Check sheet for the drawn part. Datum: minimum x, y, z corner. Units: mm. A direction names the side the tool comes from. Coordinates: 2 decimals unless noted, no trailing zeros. Order: outer loops, then holes, each group sorted by start corner. A loop starts at its lowest first (then second) coordinate and runs counter-clockwise, first axis right, second up. Notation, with made-up numbers: (12.5, -24) - (64.5, -24) arc R24 cw to (64.5, -11) - close; hole circle Ø2 at (25, 77). An arc over 180 degrees is marked (long way). Answer as CSV lines item,"result". Start each with the question number.
1. Section check A-A (y = 4.9). Record the cut outline in (x, z).
2. Mould release check, pull along Z, two halves, no side actions. Record for the marked faces 4, 5 and 6: pulls with the +Z half, pulls with the -Z half, needs draft (parallel to the pull), parting line crosses it, or undercut.
3. Material ranges on L1, parallel to Z at x = 6.5, y = 4.35; L2, parallel to Z at x = 5.5, y = 5.1; L3, parallel to Z at x = 6.5, y = 3.85, recorded low to high. Write a range as [from, to].
4. Go/stop test with a flat-tipped pin: pin 1 (2.5 mm diameter, centred on x = 7, z = 8, fed in from -Y). Record where the tip stops, or that it passes through.
5. Set-up check for the marked faces 1, 2 and 3: record each of +Z, -Z, +X, -X, +Y, -Y from which the full face is reachable in a straight line by a thin tool's end or side.
6. Section check D-D (x = 6.5). Record the cut outline in (y, z).
7. Section check B-B (y = 1.8). Record the cut outline in (x, z), and give its area (3 significant figures).
8. Section check C-C (z = 7.75). Record the cut outline in (x, y) (3 decimals).
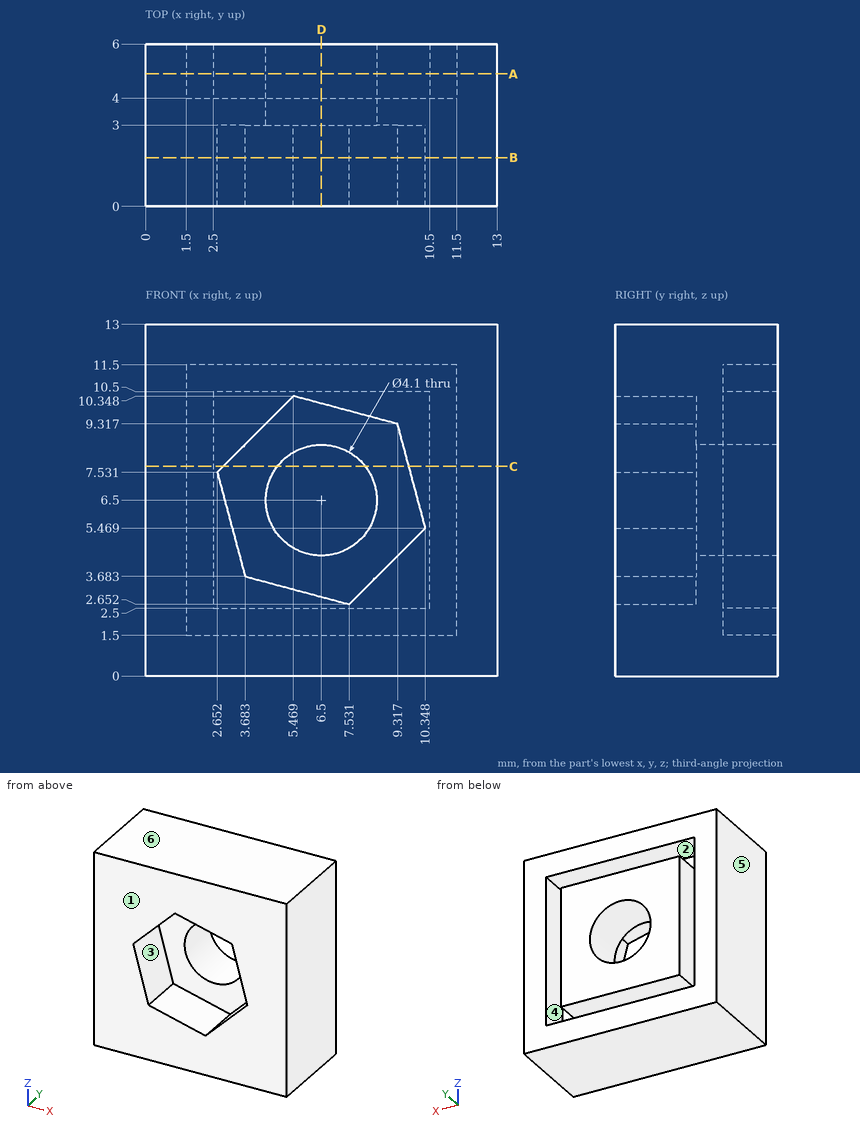
Evaluation:
1,outline,"(0, 0) - (13, 0) - (13, 13) - (0, 13) - close; (2.5, 2.5) - (10.5, 2.5) - (10.5, 10.5) - (2.5, 10.5) - close; hole (1.5, 1.5) - (11.5, 1.5) - (11.5, 11.5) - (1.5, 11.5) - close; hole circle Ø4.1 at (6.5, 6.5)"
2,face 4,"undercut"
2,face 5,"needs draft"
2,face 6,"pulls with the +Z half"
3,L1,"z = [0, 1.5], [2.5, 4.45], [8.55, 10.5], [11.5, 13]"
3,L2,"z = [0, 1.5], [2.5, 4.71], [8.29, 10.5], [11.5, 13]"
3,L3,"z = [0, 4.45], [8.55, 13]"
4,pin 1,"stops at y = 3"
5,face 1,"+Z, -Z, +X, -X, -Y"
5,face 2,"+Y"
5,face 3,"-Y"
6,outline,"(0, 0) - (6, 0) - (6, 1.5) - (4, 1.5) - (4, 2.5) - (6, 2.5) - (6, 4.45) - (3, 4.45) - (3, 2.93) - (0, 2.93) - close; (0, 10.07) - (3, 10.07) - (3, 8.55) - (6, 8.55) - (6, 10.5) - (4, 10.5) - (4, 11.5) - (6, 11.5) - (6, 13) - (0, 13) - close"
7,outline,"(0, 0) - (13, 0) - (13, 13) - (0, 13) - close; hole (2.65, 7.53) - (3.68, 3.68) - (7.53, 2.65) - (10.35, 5.47) - (9.32, 9.32) - (5.47, 10.35) - close"
7,area,"128 mm²"
8,outline,"(0, 0) - (2.871, 0) - (2.871, 3) - (4.875, 3) - (4.875, 6) - (2.5, 6) - (2.5, 4) - (1.5, 4) - (1.5, 6) - (0, 6) - close; (8.125, 3) - (9.737, 3) - (9.737, 0) - (13, 0) - (13, 6) - (11.5, 6) - (11.5, 4) - (10.5, 4) - (10.5, 6) - (8.125, 6) - close"
